Source: CAD feature listing. Evaluate the final solid. Frame: model axes, mm. A direction names the side the tool comes from. Round coordinates to 2 decimals unless told otherwise and drop trailing zeros. Write each loop counter-clockwise with the first axis right and the second up, starting at its lowest first coordinate (ties: lowest second). Pieces come first, ordered by that corner, then holes. Notation, with made-up numbers: M 71,25 L 91,25 A32 ccw 91,54 Z; hole C -39.5,61.5 d2. An arc over 180 degrees is marked long. Use a Markdown table: item, result.
```python
from build123d import *

# Parameters (mm, degrees)
SKETCH1_R               = 5.1
SKETCH1_R_2             = 4
BOSS_EXTRUDE1_DEPTH     = 1.5
SKETCH2_R               = 11
SKETCH2_R_2             = 4
BOSS_EXTRUDE2_DEPTH     = 3.5
SKETCH3_R               = 5.1
SKETCH3_R_2             = 4
BOSS_EXTRUDE3_DEPTH     = 15
CUT_EXTRUDE1_DEPTH      = 21.597329924
CUT_EXTRUDE1_DEPTH_BACK = 21.597329924
SKETCH4_R               = 1.5
CHAMFER1_SIZE           = 0.2


with BuildPart() as part:
    # Sketch1 → Boss-Extrude1 (new body)
    with BuildSketch(Plane.XY):
        Circle(SKETCH1_R)
        Circle(SKETCH1_R_2, mode=Mode.SUBTRACT)
    extrude(amount=BOSS_EXTRUDE1_DEPTH)

    # Sketch2 → Boss-Extrude2 (add)
    with BuildSketch(Plane.XY.offset(1.5)):
        Circle(SKETCH2_R)
        Circle(SKETCH2_R_2, mode=Mode.SUBTRACT)
    extrude(amount=BOSS_EXTRUDE2_DEPTH)

    # Sketch3 → Boss-Extrude3 (add)
    with BuildSketch(Plane(origin=(0, 0, 0), x_dir=(-1, 0, 0), z_dir=(0, 0, -1))):
        with Locations(Location((0, 0, 0), (0, 0, 180))):
            Circle(SKETCH3_R)
        Circle(SKETCH3_R_2, mode=Mode.SUBTRACT)
    extrude(amount=-BOSS_EXTRUDE3_DEPTH)

    # Sketch4 → Cut-Extrude1 (cut, two sides: drawn at the far end of the back side and taken through both)
    with BuildSketch(Plane(origin=(0, 0, 1.5), x_dir=(-1, 0, 0), z_dir=(0, 0, -1)).offset(-CUT_EXTRUDE1_DEPTH_BACK)):
        with Locations(Location((0, 8, 0), (0, 0, 180))):
            Circle(SKETCH4_R)
        with Locations(Location((8, 0, 0), (0, 0, 180))):
            Circle(SKETCH4_R)
        with Locations(Location((0, -8, 0), (0, 0, 180))):
            Circle(SKETCH4_R)
        with Locations(Location((-8, 0, 0), (0, 0, 180))):
            Circle(SKETCH4_R)
    extrude(amount=CUT_EXTRUDE1_DEPTH + CUT_EXTRUDE1_DEPTH_BACK, mode=Mode.SUBTRACT)

    # Chamfer1
    chamfer1_edges = [part.edges().sort_by_distance(p)[0] for p in [
        (-11, 0, 5),
        (-11, 0, 1.5),
        (-5.1, 0, 15),
        (-5.1, 0, 0),
    ]]
    chamfer(chamfer1_edges, length=CHAMFER1_SIZE)


solid = part.part
```
Q1. Section B-B on z = 9.75. Return loops of the section in (x, y), plus the area to 3 significant figures.
Results are:
| item | result |
|---|---|
| outline | C 0,0 d10.2; hole C 0,0 d8 |
| area | 31.4 mm^2 |
Q2. Mould query, pull axis X, two halves, no side actions, for faces 4 (the cylindrical face through (-2.38, -10.74, 3.23)), 5 (the cylindrical face through (6.5, -0.07, 3.27)), 6 (the flat face through (-2, 4, 15)). Classes: +X half, -X half, draft (parallel to the pull), parting line (faces both ways), or undercut.
Results are:
| item | result |
|---|---|
| face 4 | parting line |
| face 5 | undercut |
| face 6 | draft |
Q3. First-contact query: pin 1 Ø5 at (y, z) = (6.5, 9.5) entering from -X; pin 2 Ø5 at (x, y) = (0, 8) entering from -Z; pin 3 Ø8 at (x, z) = (-5, 9.5) entering from +Y. Flat tips, straight axial feed; report the tip coordinate or a pass-through.
Results are:
| item | result |
|---|---|
| pin 1 | x = -3.16 |
| pin 2 | z = 1.5 |
| pin 3 | y = 5 |
Q4. Line query: L1, parallel to Y at x = 0, z = 3.25; L2, parallel to Y at x = -8, z = 4.1; L3, parallel to Z at x = 5.5, y = -5. Output: solid intervals per line, ascending.
Results are:
| item | result |
|---|---|
| L1 | -11 to -9.5, -6.5 to -4, 4 to 6.5, 9.5 to 11 |
| L2 | -7.55 to -1.5, 1.5 to 7.55 |
| L3 | 1.5 to 5 |
Q5. Reachability of faces 1 (the flat face through (5, -2, 5)), 2 (the cylindrical face through (2.4, -4.5, 0.8)), 3 (the cylindrical face through (-9.5, -0.07, 3.27)) from +Z, -Z, +X, -X, +Y, -Y: full face, straight path, thin tool, end or side. Return the list, or none.
Results are:
| item | result |
|---|---|
| face 1 | +Z |
| face 2 | -Z |
| face 3 | +Z, -Z |
Q6. Section A-A on x = 0. Give the number of separate pieces and of enclosed holes in the cut face, plus the area to 3 significant figures.
Results are:
| item | result |
|---|---|
| separate pieces | 4 |
| enclosed holes | 0 |
| area | 53.1 mm^2 |
